Design review of the part built by this model. Coordinates are the model's own, in mm. Face numbers are marked on the shaded views. A direction names the side the tool comes from. Coordinates: 2 decimals unless noted, no trailing zeros. Write each loop counter-clockwise with the first axis right and the second up, starting at its lowest first coordinate (ties: lowest second). Pieces come first, ordered by that corner, then holes.
Q1. Take a section at D-D, the plane z = 1.7. Write out the cut boundary in (x, y) (3 decimals), plus the area to 3 significant figures.
Q2. For the marked faces 4, 5 and 6, list the 3-axis set-ups (+Z, -Z, +X, -X, +Y, -Y) from which the entire face can be reached by the end or side of a thin tool; tool diameter is ignored.
Q3. For pin 1 Ø2.5 at (x, y) = (24, 0) entering from +Z; pin 2 Ø1.8 at (x, z) = (5, 0) entering from +Y; pin 3 Ø1.2 at (x, z) = (20, 3) entering from +Y, all flat-tipped, find the tip position at first contact; note any pin that passes through.
Q4. The part is to be moulded in two halves that separate along X. For the marked faces 1, 2 and 3, say which applies: released by +X, released by -X, zero draft, split by the parting line, or undercut.
Q5. For L1, parallel to Y at x = 24, z = 2.6; L2, parallel to X at y = -1, z = 1.2; L3, parallel to Z at x = 12, y = 0.5, list the stretches that pass through material, from the lowest coordinate up.
Q6. Take a section at C-C, the plane y = 0. Write out the cut boundary in (x, z), plus the area to 3 significant figures.
Q7. Take a section at A-A, the plane z = -0.45. Write out the cut boundary in (x, y).
Q8. Take a section at B-B, the plane x = 0. Write out the cut boundary in (y, z) (3 decimals).
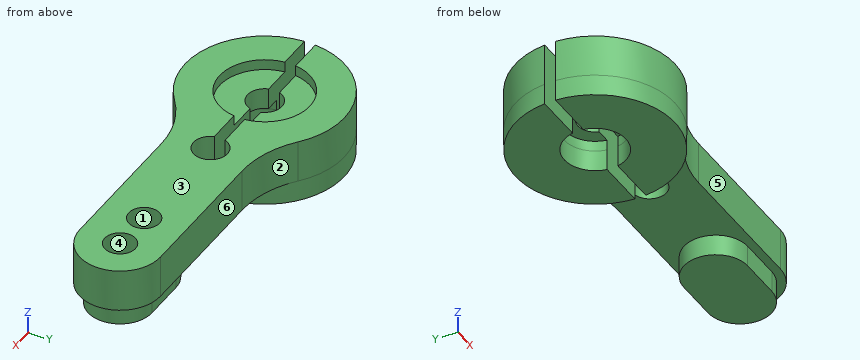
from build123d import *

# Parameters (mm, degrees)
SKETCH1_R           = 1.45
BOSS_EXTRUDE1_DEPTH = 4
BOSS_EXTRUDE3_START = 2
BOSS_EXTRUDE3_DEPTH = 2
SKETCH4_R           = 4.25
CUT_EXTRUDE1_DEPTH  = 1
SKETCH6_R           = 2.9
CUT_EXTRUDE2_DEPTH  = 1


with BuildPart() as part:
    # Sketch1 → Boss-Extrude1 (new body)
    with BuildSketch(Plane(origin=(0, 0, 0), x_dir=(0, 1, 0), z_dir=(0, 0, 1))):
        with BuildLine():
            ThreePointArc((-5.826821987, -4.722091224), (-4.321683338, -7.407935145), (-3.8, -10.442246667))
            Line((-3.8, -10.442246667), (-3.8, -24))
            ThreePointArc((-3.8, -24), (0, -27.8), (3.8, -24))
            Line((3.8, -24), (3.8, -10.442246667))
            ThreePointArc((3.8, -10.442246667), (4.321683338, -7.407935145), (5.826821987, -4.722091224))
            ThreePointArc((5.826821987, -4.722091224), (6.875471927, 2.99631203), (0.507973157, 7.482777778))
            Line((0.507973157, 7.482777778), (0.507973157, 1.543563498))
            ThreePointArc((0.507973157, 1.543563498), (1.625, 0), (0.507973157, -1.543563498))
            Line((0.507973157, -1.543563498), (0.507973157, -7.482777778))
            ThreePointArc((0.507973157, -7.482777778), (0, -10.6), (-0.507973157, -7.482777778))
            Line((-0.507973157, -7.482777778), (-0.507973157, -1.543563498))
            ThreePointArc((-0.507973157, -1.543563498), (-1.625, 0), (-0.507973157, 1.543563498))
            Line((-0.507973157, 1.543563498), (-0.507973157, 7.482777778))
            ThreePointArc((-0.507973157, 7.482777778), (-6.875471927, 2.99631203), (-5.826821987, -4.722091224))
        make_face()
        with Locations(Location((0, -24, 0), (0, 0, 270))):
            Circle(SKETCH1_R, mode=Mode.SUBTRACT)
        with Locations(Location((0, -20, 0), (0, 0, 270))):
            Circle(SKETCH1_R, mode=Mode.SUBTRACT)
    extrude(amount=BOSS_EXTRUDE1_DEPTH)

    # Sketch3 → Boss-Extrude3 (add)
    with BuildSketch(Plane(origin=(0, 0, 0), x_dir=(1, 0, 0), z_dir=(0, 0, -1)).offset(BOSS_EXTRUDE3_START)):
        with BuildLine():
            Line((20, 3), (24, 3))
            ThreePointArc((24, 3), (27, 0), (24, -3))
            Line((24, -3), (20, -3))
            ThreePointArc((20, -3), (17, 0), (20, 3))
        make_face()
        with BuildLine():
            Line((-7.482777778, 0.507973157), (-2.855164316, 0.507973157))
            ThreePointArc((-2.855164316, 0.507973157), (0, 2.9), (2.855164316, 0.507973157))
            Line((2.855164316, 0.507973157), (7.482777778, 0.507973157))
            ThreePointArc((7.482777778, 0.507973157), (0, 7.5), (-7.482777778, 0.507973157))
        make_face()
        with BuildLine():
            Line((-2.855164316, -0.507973157), (-7.482777778, -0.507973157))
            ThreePointArc((-7.482777778, -0.507973157), (0, -7.5), (7.482777778, -0.507973157))
            Line((7.482777778, -0.507973157), (2.855164316, -0.507973157))
            ThreePointArc((2.855164316, -0.507973157), (0, -2.9), (-2.855164316, -0.507973157))
        make_face()
    extrude(amount=-BOSS_EXTRUDE3_DEPTH)

    # Sketch4 → Cut-Extrude1 (cut)
    with BuildSketch(Plane.XY.offset(4)):
        Circle(SKETCH4_R)
    extrude(amount=-CUT_EXTRUDE1_DEPTH, mode=Mode.SUBTRACT)

    # Sketch6 → Cut-Extrude2 (cut)
    with BuildSketch(Plane(origin=(0, 0, 0), x_dir=(1, 0, 0), z_dir=(0, 0, -1))):
        Circle(SKETCH6_R)
    extrude(amount=-CUT_EXTRUDE2_DEPTH, mode=Mode.SUBTRACT)


solid = part.part
Responses:
1. outline: (-7.483, -0.508) arc R7.5 ccw to (4.722, -5.827) arc R9.085 cw to (10.442, -3.8) - (24, -3.8) arc R3.8 ccw to (24, 3.8) - (10.442, 3.8) arc R9.085 cw to (4.722, 5.827) arc R7.5 ccw to (-7.483, 0.508) - (-1.544, 0.508) arc R1.625 cw to (1.544, 0.508) - (7.483, 0.508) arc R1.6 cw (long way) to (7.483, -0.508) - (1.544, -0.508) arc R1.625 cw to (-1.544, -0.508) - close; hole circle Ø2.9 at (20, 0); hole circle Ø2.9 at (24, 0)
1. area: 289 mm2
2. face 4: +Z
2. face 5: +Z, -Z, +X, -Y
2. face 6: +Z, -Z, +X, +Y
3. pin 1: stops at z = 0
3. pin 2: stops at y = 6.28
3. pin 3: stops at y = 3.8
4. face 1: undercut
4. face 2: released by +X
4. face 3: zero draft
5. L1: y = -3.8 to -1.45, 1.45 to 3.8
5. L2: x = -7.43 to -1.28, 1.28 to 7.75, 10.25 to 18.95, 21.05 to 22.95, 25.05 to 27.67
5. L3: z = 0 to 4
6. outline: (10.6, 0) - (17, 0) - (17, -2) - (27, -2) - (27, 0) - (27.8, 0) - (27.8, 4) - (25.45, 4) - (25.45, 0) - (22.55, 0) - (22.55, 4) - (21.45, 4) - (21.45, 0) - (18.55, 0) - (18.55, 4) - (10.6, 4) - close
6. area: 65.6 mm2
7. outline: (-7.48, -0.51) arc R7.5 ccw to (7.48, -0.51) - (2.86, -0.51) arc R2.9 cw to (-2.86, -0.51) - close; (-7.48, 0.51) - (-2.86, 0.51) arc R2.9 cw to (2.86, 0.51) - (7.48, 0.51) arc R7.5 ccw to start; (20, -3) - (24, -3) arc R3 ccw to (24, 3) - (20, 3) arc R3 ccw to start
8. outline: (-7.5, -2) - (-2.9, -2) - (-2.9, 1) - (-1.625, 1) - (-1.625, 3) - (-4.25, 3) - (-4.25, 4) - (-7.5, 4) - close; (1.625, 1) - (2.9, 1) - (2.9, -2) - (7.5, -2) - (7.5, 4) - (4.25, 4) - (4.25, 3) - (1.625, 3) - close
